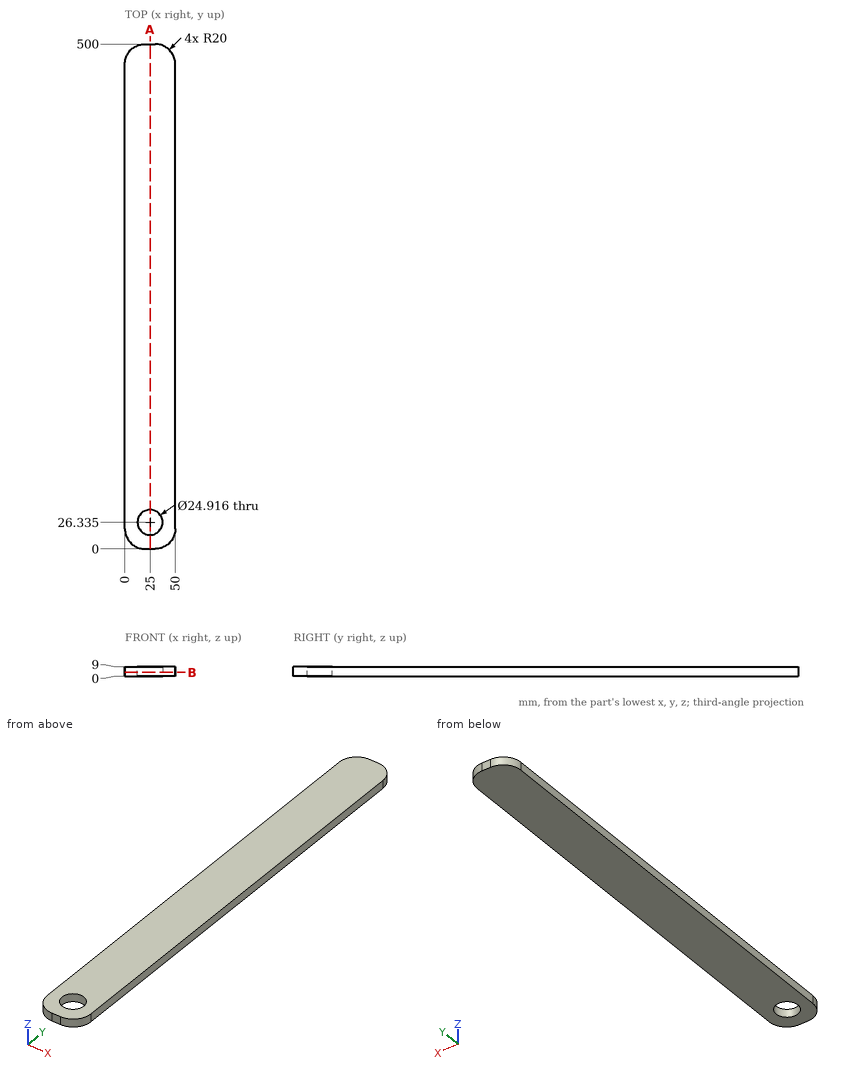
Verification items for this drawing (mm, ordinates from the low corner). Give positions to 0.01 mm unless a question says otherwise; leave off trailing zeros. Loops run counter-clockwise (first coordinate to the right, second up) from the corner with the lowest first, then second, coordinate; pieces in that order, holes last. Notation, with made-up numbers: M -1,79.5 L 38,79.5 A31 ccw 38,117.5 Z; hole C 21.5,77 d6. An arc over 180 degrees is marked long. Answer as a JSON object with one key per item and string values. Group by question number.
Q1. Cross-section at B-B on z = 3.5. Record the cut outline in (x, y) (1 decimal).
Q2. Cross-section at A-A on x = 25. Record the cut outline in (y, z).
Q3. Go/stop test with flat-tipped pins: P1, Ø1.5, axis at x = 9, z = 7, coming from the -Y side; P2, Ø20, axis at x = 25, y = 26.33, coming from the -Z side. Record where each tip stops, or that it passes through.
Q4. Material ranges on line 1 along Y through (x, z) = (25, 3.5); line 2 along Y through (x, z) = (30.5, 8) (1 decimal); line 3 along X through (y, z) = (29, 3.5), recorded low to high. Write a range as [from, to].
Evaluation:
{
 "1": {"outline": "M 0,20 A20 ccw 20,0 L 30,0 A20 ccw 50,20 L 50,480 A20 ccw 30,500 L 20,500 A20 ccw 0,480 Z; hole C 25,26.3 d24.9"},
 "2": {"outline": "M 0,0 L 13.88,0 L 13.88,9 L 0,9 Z; M 38.79,0 L 500,0 L 500,9 L 38.79,9 Z"},
 "3": {"P1": "stops at y = 2.83", "P2": "passes through"},
 "4": {"line 1": "y = [0, 13.88], [38.79, 500]", "line 2": "y = [0, 15.2], [37.5, 500]", "line 3": "x = [0, 12.83], [37.17, 50]"}
}
